Part print with two shaded views. Sizes in mm from the minimum x, y, z corner. Round coordinates to 2 decimals unless told otherwise and drop trailing zeros. Loops run counter-clockwise (first coordinate to the right, second up) from the corner with the lowest first, then second, coordinate; pieces in that order, holes last.
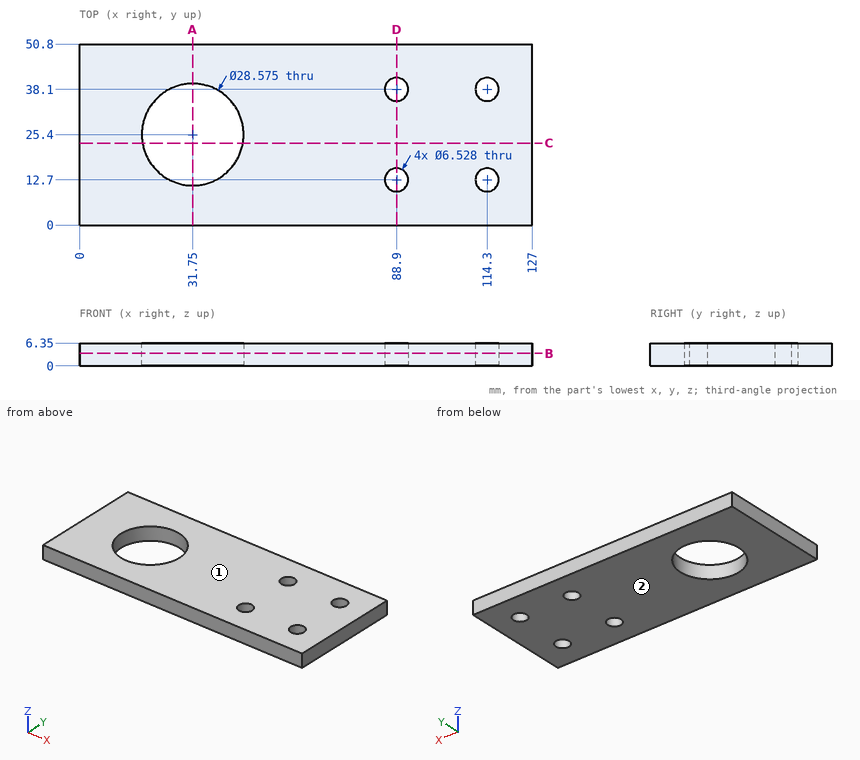
Item 1: Cut at C-C (y = 23). List the corners of the cut face in (x, z).
Verdict:
outline: (0, 0) - (17.67, 0) - (17.67, 6.35) - (0, 6.35) - close; (45.83, 0) - (127, 0) - (127, 6.35) - (45.83, 6.35) - close
Item 2: Wall check: L1, parallel to Y at x = 88.9, z = 5.25; L2, parallel to Y at x = 31.75, z = 2.75; L3, parallel to Y at x = 21, z = 2. Give the ranges that are in metal, low to high.
Verdict:
L1: y = 0 to 9.44, 15.96 to 34.84, 41.36 to 50.8
L2: y = 0 to 11.11, 39.69 to 50.8
L3: y = 0 to 15.99, 34.81 to 50.8
Item 3: Mould opens along Z. For the marked faces 1 and 2 say: released by +Z, released by -Z, zero draft, split by the parting line, or undercut.
Verdict:
face 1: released by +Z
face 2: released by -Z
Item 4: Cut at B-B (z = 3.5). State how many separate pieces and enclosed holes the cut face has, plus the area to 3 significant figures.
Verdict:
separate pieces: 1
enclosed holes: 5
area: 5,680 mm2
Item 5: Cut at A-A (x = 31.75). List the corners of the cut face in (y, z), plus the area to 3 significant figures.
Verdict:
outline: (0, 0) - (11.11, 0) - (11.11, 6.35) - (0, 6.35) - close; (39.69, 0) - (50.8, 0) - (50.8, 6.35) - (39.69, 6.35) - close
area: 141 mm2
Item 6: Cut at D-D (x = 88.9). List the corners of the cut face in (y, z).
Verdict:
outline: (0, 0) - (9.44, 0) - (9.44, 6.35) - (0, 6.35) - close; (15.96, 0) - (34.84, 0) - (34.84, 6.35) - (15.96, 6.35) - close; (41.36, 0) - (50.8, 0) - (50.8, 6.35) - (41.36, 6.35) - close
